Work out the finished part from the listing and answer in its coordinate system (mm). Coordinates: 2 decimals unless noted, no trailing zeros. Order: outer loops, then holes, each group sorted by start corner. A loop starts at its lowest first (then second) coordinate and runs counter-clockwise, first axis right, second up.
1. Find the intervals of material crossed by probe 1 along Z at (x, y) = (1.25, 2.4); probe 2 along Z at (x, y) = (8.75, 1.05); probe 3 along X at (y, z) = (2, -39.5), in increasing order.
2. Flat-ended cylindrical pins translate along their axes: pin 1 Ø1.5 at (x, y) = (19, 1) entering from -Z; pin 2 Ø0.9 at (x, y) = (15.5, 1) entering from -Z. Find the tip coordinate at first contact, or state that the pin passes through.
3. The part is cut by section B-B, the plane z = -110. Give the vertices of the cut face in (x, y).
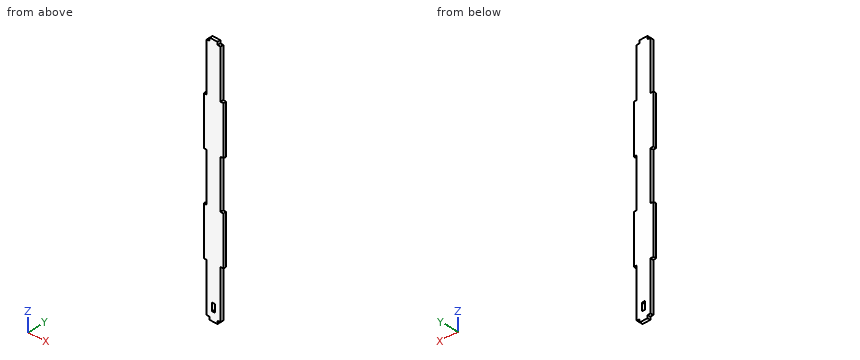
```python
from build123d import *

# Parameters (mm, degrees)
SALIENTE_EXTRUIR1_DEPTH = 3


with BuildPart() as part:
    # Croquis1 → Saliente-Extruir1 (new body)
    with BuildSketch(Plane(origin=(0, 0, 0), x_dir=(1, 0, 0), z_dir=(0, 1, 0))):
        Polygon((14, 253.116176228), (10, 253.116176228), (6, 253.116176228), (6, 250.116176228), (3, 250.116176228), (3, 200.116176228), (0, 200.116176228), (0, 150.116176228), (3, 150.116176228), (3, 100.116176228), (0, 100.116176228), (0, 50.116176228), (3, 50.116176228), (3, 0.116176228), (6, 0.116176228), (6, -2.883823772), (14, -2.883823772), (14, 0.116176228), (17, 0.116176228), (17, 50.116176228), (20, 50.116176228), (20, 100.116176228), (17, 100.116176228), (17, 150.116176228), (20, 150.116176228), (20, 200.116176228), (17, 200.116176228), (17, 250.116176228), (14, 250.116176228), align=None)
        Polygon((8.5, 244.116176228), (10, 244.116176228), (11.5, 244.116176228), (11.5, 236.116176228), (8.5, 236.116176228), align=None, mode=Mode.SUBTRACT)
    extrude(amount=SALIENTE_EXTRUIR1_DEPTH)


solid = part.part
```
Geometry says:
1. probe 1: z = -200.12 to -150.12, -100.12 to -50.12
1. probe 2: z = -253.12 to -244.12, -236.12 to 2.88
1. probe 3: x = 3 to 17
2. pin 1: stops at z = -200.12
2. pin 2: stops at z = -250.12
3. outline: (3, 0) - (17, 0) - (17, 3) - (3, 3) - close
